Here's how the part is built. I have some questions about the finished solid (model axes, mm). A direction names the side the tool comes from. Round coordinates to 2 decimals unless told otherwise and drop trailing zeros. Write each loop counter-clockwise with the first axis right and the second up, starting at its lowest first coordinate (ties: lowest second). Pieces come first, ordered by that corner, then holes. Notation, with made-up numbers: (-1.5, 16.25) - (16.5, 16.25) arc R11 cw to (16.5, 29.25) - close; hole circle Ø3 at (43.5, -26.5). An arc over 180 degrees is marked (long way). One line per item, written item: value. Start each with the question number.
Item 1: For P1, Ø1.5, axis at x = 0, y = 51.5, coming from the +Z side; P2, Ø1.5, axis at x = -1, y = -15, coming from the +Z side; P3, Ø1.6, axis at x = 0.5, z = 3.5, coming from the -Y side; P4, Ø1.3, axis at x = 0.5, z = -2, coming from the -Y side, each with a flat end and sliding along its axis, tell me the tip position at first contact or that it passes through.
Item 2: If I drill on line 1 (Z direction, x = 1.15, y = 47.5); line 2 (Y direction, x = 1.1, z = 5.5); line 3 (Y direction, x = -1.05, z = 7.75), over which ranges is the centre line in solid material (lowest first)?
Item 3: For faces 4 (the face through (0, -50, 3)), 5 (the face through (0, -50, -11)), 6 (the face through (0, 43, -2.7)), 7 (the face through (0, -50, 11)), 8 (the face through (0, 40, 0)), which set-ups out of +Z, -Z, +X, -X, +Y, -Y let a thin tool reach every point of the face, with its end or its side?
Item 4: Imagine slicing it at B-B, the plane y = 10. Please give me the cut outline in (x, z) (3 decimals), then the cut area to 4 significant figures.
Item 5: Imagine slicing it at A-A, the plane z = 5.75. Please give me the cut outline in (x, y) (3 decimals), then the cut area to 3 significant figures.
Item 6: Thinking about a two-plate mould opening in Z: for faces 1 (the face through (0, 53, 7)), 2 (the face through (0, 51, 10)), 3 (the face through (0, -47, -1.55)), which applies, released by +Z, released by -Z, zero draft, split by the parting line, or undercut?
```python
from build123d import *

# Parameters (mm, degrees)
F0_W     = 100
F0_H     = 25
F1_DEPTH = 1.525
F2_W     = 3
F2_H     = 6
F3_DEPTH = 3.05
F4_W     = 3.1
F4_H     = 5.5
F4_H_2   = 2.5
F4_W_2   = 1.15
F4_H_3   = 2
F4_W_3   = 5.5
F4_H_4   = 3.1
F4_W_4   = 2.5
F4_H_5   = 1.15
F4_W_5   = 2
F5_DEPTH = 3.05
F6_W     = 10
F6_H     = 3
F7_DEPTH = 3.05


with BuildPart() as f1:
    # F0 (on Right) → F1 (new body, symmetric)
    with BuildSketch(Plane.YZ):
        Rectangle(F0_W, F0_H)
    extrude(amount=F1_DEPTH, both=True)

    # F2 (on face) → F3 (join, through all)
    with BuildSketch(Plane.YZ.offset(1.525)):
        with Locations((-51.5, 7)):
            Rectangle(F2_W, F2_H)
        with Locations((-51.5, -7)):
            Rectangle(F2_W, F2_H)
        with Locations((51.5, -7)):
            Rectangle(F2_W, F2_H)
        with Locations((51.5, 7)):
            Rectangle(F2_W, F2_H)
    extrude(amount=-F3_DEPTH)

    # F4 (on face) → F5 (cut, through all)
    with BuildSketch(Plane.YZ.offset(1.525)):
        with Locations((0, 9.75)):
            Rectangle(F4_W, F4_H)
        with Locations((0, 5.75)):
            Rectangle(F4_W, F4_H_2)
        with Locations((-2.125, 5.75)):
            Rectangle(F4_W_2, F4_H_2)
        with Locations((2.125, 5.75)):
            Rectangle(F4_W_2, F4_H_2)
        with Locations((0, 3.5)):
            Rectangle(F4_W, F4_H_3)
        with Locations((-47.25, 0)):
            Rectangle(F4_W_3, F4_H_4)
        with Locations((-43.25, 0)):
            Rectangle(F4_W_4, F4_H_4)
        with Locations((-43.25, -2.125)):
            Rectangle(F4_W_4, F4_H_5)
        with Locations((-43.25, 2.125)):
            Rectangle(F4_W_4, F4_H_5)
        with Locations((-41, 0)):
            Rectangle(F4_W_5, F4_H_4)
        with Locations((43.25, 2.125)):
            Rectangle(F4_W_4, F4_H_5)
        with Locations((47.25, 0)):
            Rectangle(F4_W_3, F4_H_4)
        with Locations((43.25, 0)):
            Rectangle(F4_W_4, F4_H_4)
        with Locations((43.25, -2.125)):
            Rectangle(F4_W_4, F4_H_5)
        with Locations((41, 0)):
            Rectangle(F4_W_5, F4_H_4)
    extrude(amount=-F5_DEPTH, mode=Mode.SUBTRACT)

    # F6 (on face) → F7 (join, through all)
    with BuildSketch(Plane.YZ.offset(1.525)):
        with Locations((-25, 14)):
            Rectangle(F6_W, F6_H)
        with Locations((25, 14)):
            Rectangle(F6_W, F6_H)
    extrude(amount=-F7_DEPTH)


solid = f1.part
```
Values follow:
1. P1: stops at z = 10
1. P2: stops at z = 12.5
1. P3: stops at y = -53
1. P4: stops at y = -50
2. line 1: z = -12.5 to -1.55, 1.55 to 12.5
2. line 2: y = -53 to -2.7, 2.7 to 53
2. line 3: y = -53 to -1.55, 1.55 to 53
3. face 4: +X, -X, -Y
3. face 5: -Z, +X, -X, -Y
3. face 6: +X, -X
3. face 7: +Z, +X, -X, -Y
3. face 8: +X, -X, +Y
4. outline: (-1.525, -12.5) - (1.525, -12.5) - (1.525, 12.5) - (-1.525, 12.5) - close
4. area: 76.25 mm^2
5. outline: (-1.525, -53) - (1.525, -53) - (1.525, -2.7) - (-1.525, -2.7) - close; (-1.525, 2.7) - (1.525, 2.7) - (1.525, 53) - (-1.525, 53) - close
5. area: 307 mm^2
6. face 1: zero draft
6. face 2: released by +Z
6. face 3: undercut
